Source: CAD feature listing. Evaluate the final solid. Frame: model axes, mm. A direction names the side the tool comes from. Give positions to 0.01 mm unless a question says otherwise; leave off trailing zeros. Order: outer loops, then holes, each group sorted by start corner. A loop starts at its lowest first (then second) coordinate and runs counter-clockwise, first axis right, second up.
1) First-contact query: P1, Ø2, axis at x = -1, z = 0.5, coming from the +Y side; P2, Ø1, axis at y = -1.5, z = -0.5, coming from the +X side; P3, Ø3, axis at y = -3, z = -0.5, coming from the -X side. Flat tips, straight axial feed; report the tip coordinate or a pass-through.
2) Draft query along X for faces 1 (the face through (1.08, -3.33, -1.48)), 2 (the face through (-1.497, -0.099, -0.535)), 3 (the face through (-0.8, -3.6, 0)). Return one class per face: released by +X, released by -X, zero draft, split by the parting line, or undercut.
3) Section C-C, the plane x = 0. Return loops of the section in (y, z), plus the area to 3 significant figures.
4) Material intervals for line 1 (X direction, y = 0, z = 0.3); line 2 (Z direction, x = 2.75, y = -2.5); line 3 (Y direction, x = 0.5, z = -0.9), sorted ascending.
5) Section B-B, the plane y = 0. Return loops of the section in (x, z), plus the area to 3 significant figures.
6) Section A-A, the plane z = -1.1. Return loops of the section in (x, y), plus the area to 3 significant figures.
7) Section D-D, the plane y = 1.75. Return loops of the section in (x, z), plus the area to 3 significant figures.
8) Access query for faces 4 (the face through (3.233, 1.341, 0.986)), 5 (the face through (-2.7, 2.5, 0)), 6 (the face through (2.8, -2.4, 0)). Directions: +Z, -Z, +X, -X, +Y, -Y. A direction counts if a zero-diameter tool reaches every point of the face in a straight line with its end or side. Return the directions, or none.
Autodesk Inventor part; units mm, degrees
ref_plane "YZ Plane" through (0, 0, 0) normal (1, 0, 0) x (0, 1, 0)
ref_plane "XZ Plane" through (0, 0, 0) normal (0, 1, 0) x (-1, 0, 0)
ref_plane "XY Plane" through (0, 0, 0) normal (0, 0, 1) x (1, 0, 0)
sketch "スケッチ1" plane through (0, 0, 0) normal (0, 0, 1) x (1, 0, 0)
  line L0 (3.8535, 1.2181) -> (2.9816, -2.7282)
  line L1 (2.9816, -2.7282) -> (-0.8719, -3.9463)
  line L2 (-0.8719, -3.9463) -> (-3.8535, -1.2181)
  line L3 (-3.8535, -1.2181) -> (-2.9816, 2.7282)
  line L4 (-2.9816, 2.7282) -> (0.8719, 3.9463)
  line L5 (0.8719, 3.9463) -> (3.8535, 1.2181)
  circle A0 centre (0, 0) radius 3.5
  dimension "d0" = 8.0829
  dimension "d1" = 7
extrude "押し出し1" add sketch "スケッチ1" along normal blind 2 contours A0
extrude "押し出し2" add sketch "スケッチ1" against normal blind 3
hole "穴1" at (0, 0, 0) direction (0, 0, -1) diameter 3 end through all
hole "穴2" at (0, 0, 0) direction (0, 0, 1) diameter 3 end through all
properties part number "ナイロンナットm4" material "ステンレス鋼"
From the geometry:
1. P1: stops at y = 3.63
1. P2: stops at x = 3.36
1. P3: stops at x = -3.55
2. face 1: released by +X
2. face 2: undercut
2. face 3: zero draft
3. outline: (-3.67, -3) - (-1.5, -3) - (-1.5, 2) - (-3.5, 2) - (-3.5, 0) - (-3.67, 0) - close; (1.5, -3) - (3.67, -3) - (3.67, 0) - (3.5, 0) - (3.5, 2) - (1.5, 2) - close
3. area: 21.0 mm2
4. line 1: x = -3.5 to -1.5, 1.5 to 3.5
4. line 2: z = -3 to 0
4. line 3: y = -3.51 to -1.41, 1.41 to 3.83
5. outline: (-3.58, -3) - (-1.5, -3) - (-1.5, 2) - (-3.5, 2) - (-3.5, 0) - (-3.58, 0) - close; (1.5, -3) - (3.58, -3) - (3.58, 0) - (3.5, 0) - (3.5, 2) - (1.5, 2) - close
5. area: 20.5 mm2
6. outline: (-3.85, -1.22) - (-0.87, -3.95) - (2.98, -2.73) - (3.85, 1.22) - (0.87, 3.95) - (-2.98, 2.73) - close; hole circle Ø3 at (0, 0)
6. area: 35.4 mm2
7. outline: (-3.2, -3) - (3.27, -3) - (3.27, 0) - (3.03, 0) - (3.03, 2) - (-3.03, 2) - (-3.03, 0) - (-3.2, 0) - close
7. area: 31.5 mm2
8. face 4: +Z
8. face 5: +Z, -X, +Y
8. face 6: +Z, +X, -Y
